The model under review builds one solid part; all positions refer to its coordinate system, in mm. A direction names the side the tool comes from. Coordinates: 2 decimals unless noted, no trailing zeros. Write each loop counter-clockwise with the first axis right and the second up, starting at its lowest first coordinate (ties: lowest second). Pieces come first, ordered by that corner, then holes. Notation, with made-up numbers: (72.25, 14) - (85.25, 14) arc R20 ccw to (85.25, 45) - close; hole circle Ø4 at (62, 38.25). An arc over 180 degrees is marked (long way). Return JSON: item names as keys, results as strings. Group by question number.
(1) Tool access review of faces 4 (the face through (-2.348, 4.144, 0.171)), 5 (the face through (2.41, 4.11, 0.17)), 6 (the face through (-2.41, -4.11, 0.17)): name each direction out of +Z, -Z, +X, -X, +Y, -Y from which nothing blocks a thin tool from reaching the whole face with its end or side.
(2) For pin 1 Ø3 at (y, z) = (4.5, 2.5) entering from +X; pin 2 Ø1 at (y, z) = (-3.5, 2) entering from -X; pin 3 Ø3 at (y, z) = (-3.5, -2) entering from -X, all flat-tipped, find the tip position at first contact; note any pin that passes through.
(3) Draft analysis for pull direction X (two halves, no side actions). For faces 1 (the face through (2, 3, 3.302)), 2 (the face through (4.27, 2.48, 3.2)), 3 (the face through (0.45, 3.425, -0.046)), state which applies: released by +X, released by -X, zero draft, split by the parting line, or undercut.
(4) To check wall thickness, follow L1, parallel to X at y = 1, z = 0.5; L2, parallel to Y at x = 3, z = -1; L3, parallel to Y at x = -2.25, z = -2.75. State the ranges of each line that lie inside material, in increasing order. Write a range as from..to.
(5) We need section A-A on z = 1. State the section outline as (x, y) points.
```python
from build123d import *

# Parameters (mm, degrees)
EXTRUDE1_DEPTH           = 3.302
SKETCH2_OUTSIDE_W        = 41.061
SKETCH2_OUTSIDE_H        = 42.534
SKETCH2_OUTSIDE_R        = 4.7625
CUT_EXTRUDE1_DEPTH       = 7.604
CUT_EXTRUDE1_TAPER       = 60
SKETCH17_R               = 6.35
EXTRUDE3_DEPTH           = 0.254
F_5_16_24_TAPPED_HOLE1_D = 6.9088


with BuildPart() as part:
    # Sketch1 → Extrude1 (new body, symmetric)
    with BuildSketch(Plane.XY):
        Polygon((4.7625, -2.749630657), (4.7625, 2.749630657), (0, 5.499261314), (-4.7625, 2.749630657), (-4.7625, -2.749630657), (0, -5.499261314), align=None)
    extrude(amount=EXTRUDE1_DEPTH, both=True)

    # Sketch2 outside → Cut-Extrude1 (cut, through all)
    with BuildSketch(Plane.XY.offset(3.302)):
        with Locations((-0.0005, 0)):
            Rectangle(SKETCH2_OUTSIDE_W, SKETCH2_OUTSIDE_H)
        Circle(SKETCH2_OUTSIDE_R, mode=Mode.SUBTRACT)
    extrude(amount=-CUT_EXTRUDE1_DEPTH, taper=CUT_EXTRUDE1_TAPER, mode=Mode.SUBTRACT)

    # Sketch17 → Extrude3 (add)
    with BuildSketch(Plane(origin=(0, 0, -3.302), x_dir=(-1, 0, 0), z_dir=(0, 0, -1))):
        Circle(SKETCH17_R)
    extrude(amount=-EXTRUDE3_DEPTH)

    # 5/16-24 Tapped Hole1 (through all)
    with Locations(Plane.XY.offset(3.302)):
        with Locations((0, 0)):
            Hole(F_5_16_24_TAPPED_HOLE1_D / 2)


solid = part.part
```
Ans:
{
 "1": {"face 4": "+Z, -X, +Y", "face 5": "+Z, +X, +Y", "face 6": "+Z, -X, -Y"},
 "2": {"pin 1": "x = 4.33", "pin 2": "x = -4.33", "pin 3": "x = -5.87"},
 "3": {"face 1": "zero draft", "face 2": "released by +X", "face 3": "undercut"},
 "4": {"L1": "-4.76..-3.31, 3.31..4.76", "L2": "-3.77..-1.71, 1.71..3.77", "L3": "-4.2..-2.62, 2.62..4.2"},
 "5": {"outline": "(-4.76, -2.75) - (0, -5.5) - (4.76, -2.75) - (4.76, 2.75) - (0, 5.5) - (-4.76, 2.75) - close; hole circle Ø6.91 at (0, 0)"}
}
